Input: part model. Units: mm. Frame: model coordinates. Round coordinates to 2 decimals unless told otherwise and drop trailing zeros. Write each loop counter-clockwise with the first axis right and the second up, starting at its lowest first coordinate (ties: lowest second). Pieces come first, ordered by that corner, then holes. Notation, with made-up numbers: (44.25, 21.5) -> (59.25, 21.5) arc R32 ccw to (59.25, 54.5) -> close; hole circle Ø11 at (79.5, 67). An arc over 180 degrees is marked (long way). Use CSV: the item, a comma, the result in double quotes.
```python
from build123d import *

# Parameters (mm, degrees)
F0_W     = 90
F0_H     = 90
F0_R     = 1.5
F0_R_2   = 3
F1_DEPTH = 4
F2_R     = 5
F4_D     = 2
F4_DEPTH = 6


with BuildPart() as f1:
    # F0 (on Top) → F1 (new body)
    with BuildSketch(Plane.XY):
        Rectangle(F0_W, F0_H)
        with Locations((-15.597129, -30)):
            Circle(F0_R, mode=Mode.SUBTRACT)
        with Locations((15.597129, -30)):
            Circle(F0_R, mode=Mode.SUBTRACT)
        with Locations((0, -4.969076)):
            Circle(F0_R_2, mode=Mode.SUBTRACT)
        with Locations((-15.597129, 1.030924)):
            Circle(F0_R, mode=Mode.SUBTRACT)
        with Locations((15.597129, 1.030924)):
            Circle(F0_R, mode=Mode.SUBTRACT)
    extrude(amount=F1_DEPTH)

    # F2
    f2_edges = [f1.edges().sort_by_distance(p)[0] for p in [
        (-45, -45, 2),
        (45, -45, 2),
        (45, 45, 2),
        (-45, 45, 2),
    ]]
    fillet(f2_edges, radius=F2_R)

    # F4
    with Locations(Plane.XY.offset(4)):
        with Locations((-25, 43), (-43, 26), (-43, 1), (-43, -24), (-25, -39), (0, -39), (25, -39), (43, -24), (43, 1), (43, 26), (25, 43), (0, 43)):
            Hole(F4_D / 2, depth=F4_DEPTH)


solid = f1.part
```
Item 1: Line query: line 1 (Y direction, x = -25, z = 2.35); line 2 (Y direction, x = -43, z = 2.15); line 3 (X direction, y = -38.5, z = 0.75). Output: solid intervals per line, ascending.
Worked answers:
line 1,"y = -45 to -40, -38 to 42, 44 to 45"
line 2,"y = -44 to -25, -23 to 0, 2 to 25, 27 to 44"
line 3,"x = -45 to -25.87, -24.13 to -0.87, 0.87 to 24.13, 25.87 to 45"
Item 2: Section query A-A on y = -30. Return the cut outline in (x, z).
Worked answers:
outline,"(-45, 0) -> (-17.1, 0) -> (-17.1, 4) -> (-45, 4) -> close; (-14.1, 0) -> (14.1, 0) -> (14.1, 4) -> (-14.1, 4) -> close; (17.1, 0) -> (45, 0) -> (45, 4) -> (17.1, 4) -> close"
Item 3: Pull-direction query (X, two-part tool) for faces 1 (the face through (-44, 43, 2)), 2 (the face through (-2.21, -2.94, 1.97)), 3 (the face through (-1, -45, 2)); classes: +X half, -X half, draft (parallel to the pull), parting line (faces both ways), or undercut.
Worked answers:
face 1,"-X half"
face 2,"undercut"
face 3,"draft"
